```python
from build123d import *

# Parameters (mm, degrees)
SM_BASE_FLANGE_1_DEPTH             = 460
SM_EDGE_FLANGE_1_STRIP_W           = 10
SM_EDGE_FLANGE_1_STRIP_H           = 1.5
SM_EDGE_FLANGE_1_STRIP_CUT_DEPTH   = 460
SM_EDGE_FLANGE_1_STRIP_2_W         = 10
SM_EDGE_FLANGE_1_STRIP_2_H         = 1.5
SM_EDGE_FLANGE_1_STRIP_CUT_2_DEPTH = 460
SM_EDGE_FLANGE_1_DEPTH             = 460
SM_EDGE_FLANGE_1_BEND_DEPTH        = 460
SM_EDGE_FLANGE_2_STRIP_W           = 10
SM_EDGE_FLANGE_2_STRIP_H           = 1.5
SM_EDGE_FLANGE_2_STRIP_CUT_DEPTH   = 460
SM_EDGE_FLANGE_2_STRIP_2_W         = 10
SM_EDGE_FLANGE_2_STRIP_2_H         = 1.5
SM_EDGE_FLANGE_2_STRIP_CUT_2_DEPTH = 460
SM_EDGE_FLANGE_2_DEPTH             = 460
SM_EDGE_FLANGE_2_BEND_DEPTH        = 460
EXTRUDE_START                      = -1.5
EXTRUDE_1_DEPTH                    = 1.5
EXTRUDE_2_DEPTH                    = 1.5


# Sheet-metal steps are written as plain solids
with BuildPart() as part:
    # 草图1 → 基体-法兰1 (new body)
    with BuildSketch(Plane.XY):
        with BuildLine():
            Line((-60, 100), (-60, 20))
            ThreePointArc((-60, 20), (-54.142135624, 5.857864376), (-40, 0))
            Line((-40, 0), (40, 0))
            Line((40, 0), (40, 1.5))
            Line((40, 1.5), (-40, 1.5))
            ThreePointArc((-40, 1.5), (-53.081475452, 6.918524548), (-58.5, 20))
            Line((-58.5, 20), (-58.5, 100))
            Line((-58.5, 100), (-60, 100))
        make_face()
    extrude(amount=SM_BASE_FLANGE_1_DEPTH)

    # 边线-法兰1 strip (across the edge) → 边线-法兰1 strip cut (cut)
    with BuildSketch(Plane(origin=(40, 1.5, 460), x_dir=(-1, 0, 0), z_dir=(0, 0, -1))):
        with Locations((-1.5, -0.75)):
            Rectangle(SM_EDGE_FLANGE_1_STRIP_W, SM_EDGE_FLANGE_1_STRIP_H)
    extrude(amount=SM_EDGE_FLANGE_1_STRIP_CUT_DEPTH, mode=Mode.SUBTRACT)

    # 边线-法兰1 strip 2 (across the edge) → 边线-法兰1 strip cut 2 (cut)
    with BuildSketch(Plane(origin=(-58.5, 100, 0), x_dir=(0, -1, 0), z_dir=(0, 0, 1))):
        with Locations((-1.5, -0.75)):
            Rectangle(SM_EDGE_FLANGE_1_STRIP_2_W, SM_EDGE_FLANGE_1_STRIP_2_H)
    extrude(amount=SM_EDGE_FLANGE_1_STRIP_CUT_2_DEPTH, mode=Mode.SUBTRACT)

    # 边线-法兰1 section (across the edge) → 边线-法兰1 (add)
    with BuildSketch(Plane(origin=(40, 1.5, 460), x_dir=(-1, 0, 0), z_dir=(0, 0, -1))):
        with BuildLine():
            Line((0, 2), (0, 13.5))
            Line((0, 13.5), (1.5, 13.5))
            Line((1.5, 13.5), (1.5, 2))
            ThreePointArc((1.5, 2), (2.085786438, 0.585786438), (3.5, 0))
            Line((3.5, 0), (3.5, -1.5))
            ThreePointArc((3.5, -1.5), (1.025126266, -0.474873734), (0, 2))
        make_face()
    extrude(amount=SM_EDGE_FLANGE_1_DEPTH)

    # 边线-法兰1 section 2 (across the edge) → 边线-法兰1 bend (add)
    with BuildSketch(Plane(origin=(-58.5, 100, 0), x_dir=(0, -1, 0), z_dir=(0, 0, 1))):
        with BuildLine():
            Line((0, 2), (0, 13.5))
            Line((0, 13.5), (1.5, 13.5))
            Line((1.5, 13.5), (1.5, 2))
            ThreePointArc((1.5, 2), (2.085786438, 0.585786438), (3.5, 0))
            Line((3.5, 0), (3.5, -1.5))
            ThreePointArc((3.5, -1.5), (1.025126266, -0.474873734), (0, 2))
        make_face()
    extrude(amount=SM_EDGE_FLANGE_1_BEND_DEPTH)

    # 边线-法兰2 strip (across the edge) → 边线-法兰2 strip cut (cut)
    with BuildSketch(Plane(origin=(38.5, 15, 460), x_dir=(0, -1, 0), z_dir=(0, 0, -1))):
        with Locations((-1.5, -0.75)):
            Rectangle(SM_EDGE_FLANGE_2_STRIP_W, SM_EDGE_FLANGE_2_STRIP_H)
    extrude(amount=SM_EDGE_FLANGE_2_STRIP_CUT_DEPTH, mode=Mode.SUBTRACT)

    # 边线-法兰2 strip 2 (across the edge) → 边线-法兰2 strip cut 2 (cut)
    with BuildSketch(Plane(origin=(-45, 98.5, 0), x_dir=(-1, 0, 0), z_dir=(0, 0, 1))):
        with Locations((-1.5, -0.75)):
            Rectangle(SM_EDGE_FLANGE_2_STRIP_2_W, SM_EDGE_FLANGE_2_STRIP_2_H)
    extrude(amount=SM_EDGE_FLANGE_2_STRIP_CUT_2_DEPTH, mode=Mode.SUBTRACT)

    # 边线-法兰2 section (across the edge) → 边线-法兰2 (add)
    with BuildSketch(Plane(origin=(38.5, 15, 460), x_dir=(0, -1, 0), z_dir=(0, 0, -1))):
        with BuildLine():
            Line((0, 2), (0, 13.5))
            Line((0, 13.5), (1.5, 13.5))
            Line((1.5, 13.5), (1.5, 2))
            ThreePointArc((1.5, 2), (2.085786438, 0.585786438), (3.5, 0))
            Line((3.5, 0), (3.5, -1.5))
            ThreePointArc((3.5, -1.5), (1.025126266, -0.474873734), (0, 2))
        make_face()
    extrude(amount=SM_EDGE_FLANGE_2_DEPTH)

    # 边线-法兰2 section 2 (across the edge) → 边线-法兰2 bend (add)
    with BuildSketch(Plane(origin=(-45, 98.5, 0), x_dir=(-1, 0, 0), z_dir=(0, 0, 1))):
        with BuildLine():
            Line((0, 2), (0, 13.5))
            Line((0, 13.5), (1.5, 13.5))
            Line((1.5, 13.5), (1.5, 2))
            ThreePointArc((1.5, 2), (2.085786438, 0.585786438), (3.5, 0))
            Line((3.5, 0), (3.5, -1.5))
            ThreePointArc((3.5, -1.5), (1.025126266, -0.474873734), (0, 2))
        make_face()
    extrude(amount=SM_EDGE_FLANGE_2_BEND_DEPTH)

    # 草图22 → 凸台-拉伸1 (add)
    with BuildSketch(Plane.XY.offset(460).offset(EXTRUDE_START)):
        with BuildLine():
            Line((-45, 96.5), (-45, 85))
            Line((-45, 85), (-45, 15))
            Line((-45, 15), (25, 15))
            Line((25, 15), (36.5, 15))
            ThreePointArc((36.5, 15), (38.974873734, 13.974873734), (40, 11.5))
            Line((40, 11.5), (40, 3.5))
            ThreePointArc((40, 3.5), (38.974873734, 1.025126266), (36.5, 0))
            Line((36.5, 0), (-40, 0))
            ThreePointArc((-40, 0), (-54.142135624, 5.857864376), (-60, 20))
            Line((-60, 20), (-60, 96.5))
            ThreePointArc((-60, 96.5), (-58.974873734, 98.974873734), (-56.5, 100))
            Line((-56.5, 100), (-48.5, 100))
            ThreePointArc((-48.5, 100), (-46.025126266, 98.974873734), (-45, 96.5))
        make_face()
    extrude(amount=EXTRUDE_1_DEPTH)

    # 草图23 → 凸台-拉伸2 (add)
    with BuildSketch(Plane(origin=(0, 0, 0), x_dir=(-1, 0, 0), z_dir=(0, 0, -1))):
        with BuildLine():
            Line((-25, 15), (45, 15))
            Line((45, 15), (45, 85))
            Line((45, 85), (45, 96.5))
            ThreePointArc((45, 96.5), (46.025126266, 98.974873734), (48.5, 100))
            Line((48.5, 100), (56.5, 100))
            ThreePointArc((56.5, 100), (58.974873734, 98.974873734), (60, 96.5))
            Line((60, 96.5), (60, 20))
            ThreePointArc((60, 20), (54.142135624, 5.857864376), (40, 0))
            Line((40, 0), (-36.5, 0))
            ThreePointArc((-36.5, 0), (-38.974873734, 1.025126266), (-40, 3.5))
            Line((-40, 3.5), (-40, 11.5))
            ThreePointArc((-40, 11.5), (-38.974873734, 13.974873734), (-36.5, 15))
            Line((-36.5, 15), (-25, 15))
        make_face()
    extrude(amount=-EXTRUDE_2_DEPTH)


solid = part.part
```
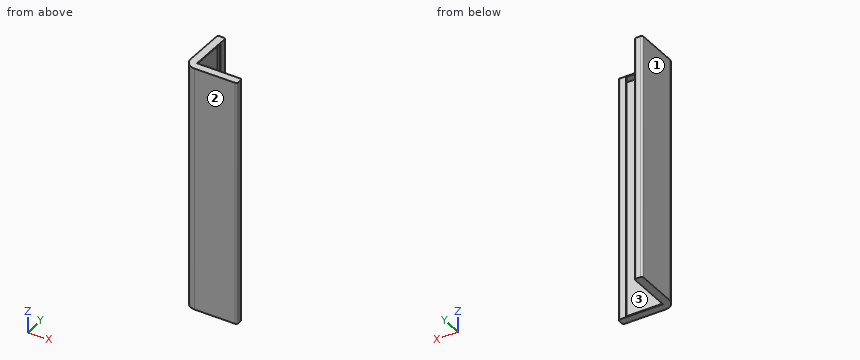
Geometry check sheet. Reference: the model listing, model coordinates, mm. Face numbers are marked on the shaded views. Give positions to 0.01 mm unless a question says otherwise; leave off trailing zeros. Loops run counter-clockwise (first coordinate to the right, second up) from the corner with the lowest first, then second, coordinate; pieces in that order, holes last. Notation, with made-up numbers: (37.5, 68.25) - (69.5, 68.25) arc R28 cw to (69.5, 103.25) - close; hole circle Ø3 at (-31, -12). An arc over 180 degrees is marked (long way). Use CSV: the item, a comma, the result in double quotes. Start each with the question number.
Q1. Section check A-A, the plane z = 321. Record the cut outline in (x, y), and give its area (3 significant figures).
Q2. Section check B-B, the plane x = -1.5. Record the cut outline in (y, z), and give its area (4 significant figures).
Q3. Go/stop test with flat-tipped pins: pin 1 Ø1.2 at (y, z) = (14, 283) entering from -X; pin 2 Ø1 at (x, z) = (-3, 64) entering from +Y; pin 3 Ø1 at (x, z) = (-43, 412.5) entering from -Y. Record where each tip stops, or that it passes through.
Q4. Section check D-D, the plane y = 57. Record the cut outline in (x, z), and give its area (4 significant figures).
Q5. Scan lines: probe 1 along Z at (x, y) = (-46, 10); probe 2 along X at (y, z) = (95, 270); probe 3 along Y at (x, z) = (-41, 176). Record each from-to range of solid material in increasing order. Write a range as from..to.
Q6. Release check for a two-part mould opening along X. For the marked faces 1, 2 and 3 record: +X half, -X half, draft (parallel to the pull), parting line (faces both ways), or undercut.
Q7. Section check C-C, the plane y = 7.5. Record the cut outline in (x, z), and give its area (3 significant figures).
Findings below:
1,outline,"(-60, 20) arc R20 ccw to (-40, 0) - (36.5, 0) arc R3.5 ccw to (40, 3.5) - (40, 11.5) arc R3.5 ccw to (36.5, 15) - (25, 15) - (25, 13.5) - (36.5, 13.5) arc R2 cw to (38.5, 11.5) - (38.5, 3.5) arc R2 cw to (36.5, 1.5) - (-40, 1.5) arc R18.5 cw to (-58.5, 20) - (-58.5, 96.5) arc R2 cw to (-56.5, 98.5) - (-48.5, 98.5) arc R2 cw to (-46.5, 96.5) - (-46.5, 85) - (-45, 85) - (-45, 96.5) arc R3.5 ccw to (-48.5, 100) - (-56.5, 100) arc R3.5 ccw to (-60, 96.5) - close"
1,area,"359 mm^2"
2,outline,"(0, 0) - (15, 0) - (15, 1.5) - (1.5, 1.5) - (1.5, 458.5) - (15, 458.5) - (15, 460) - (0, 460) - close"
2,area,"730.5 mm^2"
3,pin 1,"stops at x = -59.26"
3,pin 2,"stops at y = 1.5"
3,pin 3,"stops at y = 0.16"
4,outline,"(-60, 0) - (-45, 0) - (-45, 1.5) - (-58.5, 1.5) - (-58.5, 458.5) - (-45, 458.5) - (-45, 460) - (-60, 460) - close"
4,area,"730.5 mm^2"
5,probe 1,"z = 0..1.5, 458.5..460"
5,probe 2,"x = -60..-58.5, -46.5..-45"
5,probe 3,"y = 0.03..1.53"
6,face 1,"-X half"
6,face 2,"draft"
6,face 3,"undercut"
7,outline,"(-55.61, 0) - (40, 0) - (40, 460) - (-55.61, 460) - close; hole (-53.64, 1.5) - (38.5, 1.5) - (38.5, 458.5) - (-53.64, 458.5) - close"
7,area,"1,870 mm^2"
